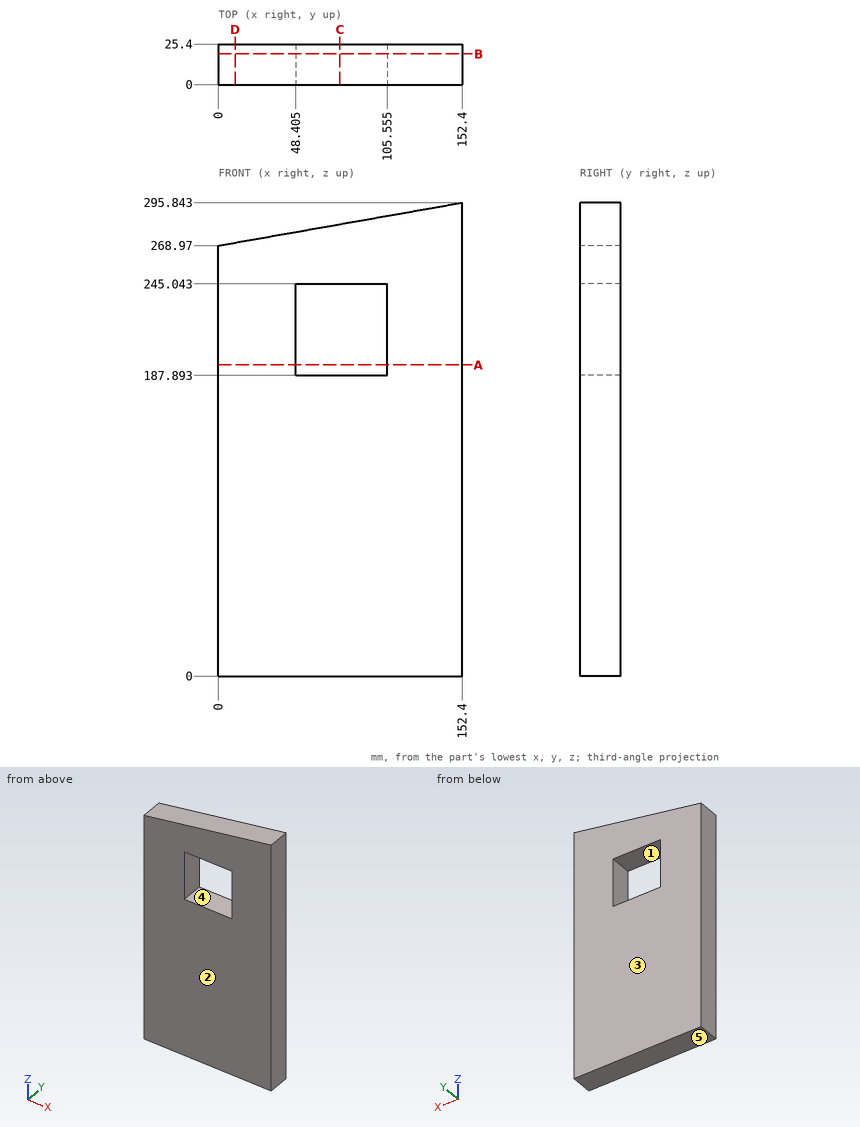
Geometry: see drawing. Coordinates: mm, zero at the bounding-box minimum. A direction names the side the tool comes from. Coordinates: 2 decimals unless noted, no trailing zeros. Order: outer loops, then holes, each group sorted by start corner. A loop starts at its lowest first (then second) coordinate and runs counter-clockwise, first axis right, second up. Notation, with made-up numbers: M 71,25.5 L 97,25.5 A21 cw 97,46.5 Z; hole C 64.25,59.25 d1. An arc over 180 degrees is marked long. Write item = value, one per line. Start each with the question number.
(1) Section D-D on x = 10.5. Output: boundary loops of the cut face in (y, z).
(2) Section C-C on x = 76. Output: boundary loops of the cut face in (y, z).
(3) Reachability of the marked faces 1 and 2 from +Z, -Z, +X, -X, +Y, -Y: full face, straight path, thin tool, end or side. Return the list, or none.
(4) First-contact query: P1, Ø12, axis at x = 107, y = 3.5, coming from the +Z side (1 decimal); P2, Ø2, axis at x = 82.5, y = 20.5, coming from the +Z side. Flat tips, straight axial feed; report the tip coordinate or a pass-through.
(5) Section A-A on z = 194.5. Output: boundary loops of the cut face in (x, y) (1 decimal), and give its area (3 significant figures).
(6) Line query: line 1 along X through (y, z) = (4, 230) (1 decimal); line 2 along Z through (x, y) = (99, 11); line 3 along Z through (x, y) = (70, 15.75). Output: solid intervals per line, ascending. Write a range as [from, to].
(7) Section B-B on y = 19.25. Output: boundary loops of the cut face in (x, z) (1 decimal), and give its area (3 significant figures).
(8) Pull-direction query (Z, two-part tool) for the marked faces 3, 4 and 5; classes: released by +Z, released by -Z, zero draft, split by the parting line, or undercut.
Result set:
q1.outline = M 0,0 L 25.4,0 L 25.4,270.82 L 0,270.82 Z
q2.outline = M 0,0 L 25.4,0 L 25.4,187.89 L 0,187.89 Z; M 0,245.04 L 25.4,245.04 L 25.4,282.37 L 0,282.37 Z
q3.face_1 = +Y, -Y
q3.face_2 = +Z, -Z, +X, -X, -Y
q4.P1 = 288.9
q4.P2 = 283.69
q5.outline = M 0,0 L 48.4,0 L 48.4,25.4 L 0,25.4 Z; M 105.6,0 L 152.4,0 L 152.4,25.4 L 105.6,25.4 Z
q5.area = 2,420 mm²
q6.line_1 = [0, 48.4], [105.6, 152.4]
q6.line_2 = [0, 187.89], [245.04, 286.43]
q6.line_3 = [0, 187.89], [245.04, 281.31]
q7.outline = M 0,0 L 152.4,0 L 152.4,295.8 L 0,269 Z; hole M 48.4,187.9 L 105.6,187.9 L 105.6,245 L 48.4,245 Z
q7.area = 39,800 mm²
q8.face_3 = zero draft
q8.face_4 = undercut
q8.face_5 = released by -Z
